Read the model definition and answer for the solid it produces. Units are mm, in the model's axes. Face numbers are marked on the shaded views. A direction names the side the tool comes from. Give positions to 0.01 mm unless a question says otherwise; leave off trailing zeros. Loops run counter-clockwise (first coordinate to the right, second up) from the corner with the lowest first, then second, coordinate; pieces in that order, holes last. Notation, with made-up numbers: (3.25, 41.5) - (10.25, 41.5) arc R26 cw to (10.25, 71.5) - close; hole circle Ø10 at (57.5, 18.5). An arc over 180 degrees is marked (long way). Put each result on its own line as item: value. Start each with the question number.
1. A cutting plane is placed at B-B, the plane x = 1. Determine the outline of the cut face in (y, z), plus the area to 3 significant figures.
2. Consider L1, parallel to Z at x = 0, y = 2.9; L2, parallel to X at y = 2.95, z = 6; L3, parallel to X at y = 2.4, z = -14. Determine where each line is inside the solid, lowest interval first. Write a range as from..to.
3. A cutting plane is placed at D-D, the plane z = 19. Determine the outline of the cut face in (x, y), plus the area to 3 significant figures.
4. A cutting plane is placed at A-A, the plane z = 0. Determine the outline of the cut face in (x, y).
5. Given pin 1 Ø2 at (y, z) = (2.5, -3) entering from -X; pin 2 Ø1.5 at (x, y) = (-5, 1.5) entering from -Z; pin 3 Ø4.5 at (x, z) = (0, -19.43) entering from -Y, each flat-ended and moving along its own axis, determine where each tip first touches the part or whether it passes through.
6. For the marked faces 1, 2 and 3, determine the directions among +Z, -Z, +X, -X, +Y, -Y from which every point of the face is accessible in a straight line to the end or side of a thin tool.
7. A cutting plane is placed at C-C, the plane y = 3.1. Determine the outline of the cut face in (x, z).
```python
from build123d import *

# Parameters (mm, degrees)
SKETCH1_R           = 4
BOSS_EXTRUDE1_DEPTH = 4
SKETCH2_R           = 1.5
CUT_EXTRUDE1_DEPTH  = 10
SKETCH3_R           = 2.5
CUT_EXTRUDE2_DEPTH  = 2
SKETCH4_R           = 10
SKETCH4_R_2         = 4
BOSS_EXTRUDE3_DEPTH = 4
FILLET1_R           = 2


with BuildPart() as part:
    # Sketch1 → Boss-Extrude1 (new body)
    with BuildSketch(Plane(origin=(0, 0, 0), x_dir=(1, 0, 0), z_dir=(0, 1, 0))):
        with BuildLine():
            Line((5.25, -21), (5.25, 21))
            ThreePointArc((5.25, 21), (4.371320344, 23.121320344), (2.25, 24))
            Line((2.25, 24), (-2.25, 24))
            ThreePointArc((-2.25, 24), (-4.371320344, 23.121320344), (-5.25, 21))
            Line((-5.25, 21), (-5.25, -21))
            ThreePointArc((-5.25, -21), (-4.371320344, -23.121320344), (-2.25, -24))
            Line((-2.25, -24), (2.25, -24))
            ThreePointArc((2.25, -24), (4.371320344, -23.121320344), (5.25, -21))
        make_face()
        with Locations((-0.25, 0)):
            Circle(SKETCH1_R, mode=Mode.SUBTRACT)
    extrude(amount=BOSS_EXTRUDE1_DEPTH)

    # Sketch2 → Cut-Extrude1 (cut)
    with BuildSketch(Plane.XZ):
        with Locations((0, 19.428521822)):
            Circle(SKETCH2_R)
        with Locations((0, -19.428521822)):
            Circle(SKETCH2_R)
    extrude(amount=-CUT_EXTRUDE1_DEPTH, mode=Mode.SUBTRACT)

    # Sketch3 → Cut-Extrude2 (cut)
    with BuildSketch(Plane.XZ):
        with Locations((0, 19.428521822)):
            Circle(SKETCH3_R)
        with Locations((0, -19.428521822)):
            Circle(SKETCH3_R)
    extrude(amount=-CUT_EXTRUDE2_DEPTH, mode=Mode.SUBTRACT)

    # Sketch4 → Boss-Extrude3 (add)
    with BuildSketch(Plane.XZ):
        with Locations((-0.25, 0)):
            Circle(SKETCH4_R)
        with Locations((-0.25, 0)):
            Circle(SKETCH4_R_2, mode=Mode.SUBTRACT)
    extrude(amount=-BOSS_EXTRUDE3_DEPTH)

    # Fillet1
    fillet1_edges = [part.edges().sort_by_distance(p)[0] for p in [
        (5.25, 0, 14.675823272),
        (4.371320344, 0, 23.121320344),
        (-5.25, 0, 14.830127019),
        (5.25, 0, -14.675823272),
        (9.75, 0, 0),
        (-10.25, 0, 0),
        (0, 0, 24),
        (-4.371320344, 0, 23.121320344),
        (-5.25, 0, -14.830127019),
        (-4.371320344, 0, -23.121320344),
        (0, 0, -24),
        (4.371320344, 0, -23.121320344),
    ]]
    fillet(fillet1_edges, radius=FILLET1_R)


solid = part.part
```
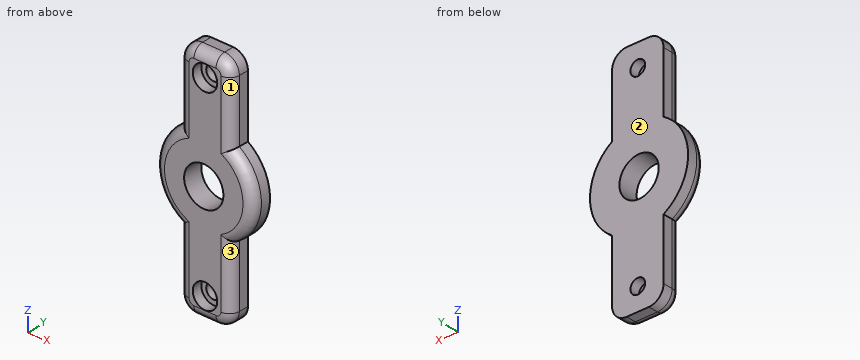
Return value:
1. outline: (0, -22) arc R2 ccw to (2, -24) - (4, -24) - (4, -20.55) - (2, -20.55) - (2, -21.72) - (0, -21.72) - close; (0, -17.14) - (2, -17.14) - (2, -18.31) - (4, -18.31) - (4, -3.8) - (0, -3.8) - close; (0, 3.8) - (4, 3.8) - (4, 18.31) - (2, 18.31) - (2, 17.14) - (0, 17.14) - close; (0, 21.72) - (2, 21.72) - (2, 20.55) - (4, 20.55) - (4, 24) - (2, 24) arc R2 ccw to (0, 22) - close
1. area: 133 mm2
2. L1: z = -24..-20.93, -17.93..-3.99, 3.99..17.93, 20.93..24
2. L2: x = -8.25..7.75
2. L3: x = -5.25..5.25
3. outline: (-5.25, 2) arc R2 ccw to (-3.25, 0) - (-2.46, 0) - (-2.46, 2) - (-1.44, 2) - (-1.44, 4) - (-5.25, 4) - close; (1.44, 2) - (2.46, 2) - (2.46, 0) - (3.25, 0) arc R2 ccw to (5.25, 2) - (5.25, 4) - (1.44, 4) - close
3. area: 24.7 mm2
4. outline: (-10.25, 2) arc R2 ccw to (-8.25, 0) - (-4.25, 0) - (-4.25, 4) - (-10.25, 4) - close; (3.75, 0) - (7.75, 0) arc R2 ccw to (9.75, 2) - (9.75, 4) - (3.75, 4) - close
5. pin 1: stops at x = -10.05
5. pin 2: stops at z = -23.18
5. pin 3: stops at y = 2
6. face 1: +Z, +X, -Y
6. face 2: +Z, -Z, +X, -X, +Y
6. face 3: -Z, +X, -Y
7. outline: (-5.25, -21) arc R3 ccw to (-2.25, -24) - (2.25, -24) arc R3 ccw to (5.25, -21) - (5.25, -8.35) arc R10 ccw to (5.25, 8.35) - (5.25, 21) arc R3 ccw to (2.25, 24) - (-2.25, 24) arc R3 ccw to (-5.25, 21) - (-5.25, 8.66) arc R10 ccw to (-5.25, -8.66) - close; hole circle Ø8 at (-0.25, 0); hole circle Ø3 at (0, -19.43); hole circle Ø3 at (0, 19.43)
